from build123d import *

# Parameters (mm, degrees)
SKETCH1_W               = 22.86
SKETCH1_H               = 20.955
BOSS_EXTRUDE1_DEPTH     = 10.4775
CUT_EXTRUDE1_DEPTH      = 33.733310729
CUT_EXTRUDE1_DEPTH_BACK = 33.733310729
CUT_EXTRUDE2_DEPTH      = 33.733310729
SKETCH4_R               = 7.9375
BOSS_EXTRUDE2_DEPTH     = 35.56
SKETCH5_R               = 4.7625
CUT_EXTRUDE3_DEPTH      = 31.242
FILLET1_R               = 2.54
CHAMFER1_SIZE           = 1.27


with BuildPart() as part:
    # Sketch1 → Boss-Extrude1 (new, symmetric)
    with BuildSketch(Plane(origin=(0, 0, 0), x_dir=(1, 0, 0), z_dir=(0, 1, 0))):
        with Locations((11.43, 0)):
            Rectangle(SKETCH1_W, SKETCH1_H)
    extrude(amount=BOSS_EXTRUDE1_DEPTH, both=True)

    # Sketch2 → Cut-Extrude1 (cut, two sides: drawn at the far end of the back side and taken through both)
    with BuildSketch(Plane(origin=(0, 10.4775, 0), x_dir=(1, 0, 0), z_dir=(0, 1, 0)).offset(-CUT_EXTRUDE1_DEPTH_BACK)):
        with BuildLine():
            Line((2.921, 3.7338), (2.921, -3.7338))
            ThreePointArc((2.921, -3.7338), (4.036923164, -6.427876836), (6.731, -7.5438))
            Line((6.731, -7.5438), (22.86, -7.5438))
            Line((22.86, -7.5438), (22.86, 7.5438))
            Line((22.86, 7.5438), (6.731, 7.5438))
            ThreePointArc((6.731, 7.5438), (4.036923164, 6.427876836), (2.921, 3.7338))
        make_face()
    extrude(amount=CUT_EXTRUDE1_DEPTH + CUT_EXTRUDE1_DEPTH_BACK, mode=Mode.SUBTRACT)

    # Sketch3 → Cut-Extrude2 (cut, through all)
    with BuildSketch(Plane.XY.offset(10.4775)):
        with BuildLine():
            ThreePointArc((16.951908562, 7.673682763), (21.211869472, 4.842286433), (22.86, 0))
            Line((22.86, 0), (22.86, 10.4775))
            Line((22.86, 10.4775), (6.35, 10.4775))
            Line((6.35, 10.4775), (16.951908562, 7.673682763))
        make_face()
        with BuildLine():
            Line((22.86, -10.4775), (22.86, 0))
            ThreePointArc((22.86, 0), (21.211869472, -4.842286433), (16.951908562, -7.673682763))
            Line((16.951908562, -7.673682763), (6.35, -10.4775))
            Line((6.35, -10.4775), (22.86, -10.4775))
        make_face()
        with BuildLine():
            ThreePointArc((18.0975, 0), (14.9225, 3.175), (11.7475, 0))
            Line((11.7475, 0), (18.0975, 0))
        make_face()
        with BuildLine():
            Line((18.0975, 0), (11.7475, 0))
            ThreePointArc((11.7475, 0), (14.9225, -3.175), (18.0975, 0))
        make_face()
    extrude(amount=-CUT_EXTRUDE2_DEPTH, mode=Mode.SUBTRACT)

    # Sketch4 → Boss-Extrude2 (add)
    with BuildSketch(Plane.ZY):
        with Locations(Location((0, 0, 0), (0, 0, 180))):
            Circle(SKETCH4_R)
    extrude(amount=BOSS_EXTRUDE2_DEPTH)

    # Sketch5 → Cut-Extrude3 (cut)
    with BuildSketch(Plane.ZY.offset(35.56)):
        Circle(SKETCH5_R)
    extrude(amount=-CUT_EXTRUDE3_DEPTH, mode=Mode.SUBTRACT)

    # Fillet1
    fillet1_edges = [part.edges().sort_by_distance(p)[0] for p in [
        (0, 0, 7.9375),
    ]]
    fillet(fillet1_edges, radius=FILLET1_R - 0.0001)  # a hair under: the kernel refuses the full size

    # Chamfer1
    chamfer1_edges = [part.edges().sort_by_distance(p)[0] for p in [
        (-35.56, 0, 7.9375),
    ]]
    chamfer(chamfer1_edges, length=CHAMFER1_SIZE)


solid = part.part
Verification items for the finished model (mm, model axes). A direction names the side the tool comes from. Give positions to 0.01 mm unless a question says otherwise; leave off trailing zeros. Loops run counter-clockwise (first coordinate to the right, second up) from the corner with the lowest first, then second, coordinate; pieces in that order, holes last.
1. Go/stop test with flat-tipped pins: P1, Ø7.5, axis at y = 0, z = 0, coming from the +X side; P2, Ø4, axis at y = 3.5, z = -6.5, coming from the +X side; P3, Ø1, axis at y = 7, z = 5.5, coming from the +X side; P4, Ø4, axis at x = 14.92, y = 0, coming from the +Z side. Record where each tip stops, or that it passes through.
Derived:
P1: stops at x = 2.92
P2: stops at x = 22.65
P3: stops at x = 3.67
P4: passes through
2. Cross-section at B-B on x = 19.5. Record the cut outline in (y, z), and give its area (3 significant figures).
Derived:
outline: (-6.48, -10.48) - (6.48, -10.48) - (6.48, -7.54) - (-6.48, -7.54) - close; (-6.48, 7.54) - (6.48, 7.54) - (6.48, 10.48) - (-6.48, 10.48) - close
area: 76.1 mm2
3. Tool access check on faces 5 (the flat face through (9, 0, 10.478)), 6 (the cylindrical face through (4.07, -0.15, -6.46)), 7 (the cylindrical face through (-20.16, -2.9, -3.78)). Record the directions out of +Z, -Z, +X, -X, +Y, -Y that give a thin tool (end or side, any length) a straight path to the whole face; none if there is none.
Derived:
face 5: +Z, +X, -X, +Y, -Y
face 6: +X, +Y, -Y
face 7: -X
4. Cross-section at D-D on x = -14. Record the cut outline in (y, z) (1 decimal).
Derived:
outline: circle Ø15.9 at (0, 0); hole circle Ø9.5 at (0, 0)
5. Cross-section at A-A on x = 13.5. Record the cut outline in (y, z), and give its area (3 significant figures).
Derived:
outline: (-8.59, -10.48) - (-2.84, -10.48) - (-2.84, -7.54) - (-8.59, -7.54) - close; (-8.59, 7.54) - (-2.84, 7.54) - (-2.84, 10.48) - (-8.59, 10.48) - close; (2.84, -10.48) - (8.59, -10.48) - (8.59, -7.54) - (2.84, -7.54) - close; (2.84, 7.54) - (8.59, 7.54) - (8.59, 10.48) - (2.84, 10.48) - close
area: 67.5 mm2
6. Material ranges on probe 1 along Z at (x, y) = (13, 6.25); probe 2 along Y at (x, z) = (-11, 0); probe 3 along X at (y, z) = (-1.25, 0), recorded low to high.
Derived:
probe 1: z = -10.48 to -7.54, 7.54 to 10.48
probe 2: y = -7.94 to -4.76, 4.76 to 7.94
probe 3: x = -4.32 to 2.92
7. Release check for a two-part mould opening along Y. For faces 1 (the cylindrical face through (17.26, -2.15, -8.99)), 2 (the flat face through (11, 0, 7.544)), 3 (the flat face through (2, -10.478, 0)), 4 (the flat face through (2, 10.478, 0)) record: +Y half, -Y half, draft (parallel to the pull), parting line (faces both ways), or undercut.
Derived:
face 1: undercut
face 2: draft
face 3: -Y half
face 4: +Y half
